```python
from build123d import *

# Parameters (mm, degrees)
SKETCH1_W                       = 150
SKETCH1_H                       = 55
BOSS_EXTRUDE1_DEPTH             = 19.6
SKETCH2_W                       = 27.5
SKETCH2_H                       = 55
BOSS_EXTRUDE2_DEPTH             = 19.6
M8_CLEARANCE_HOLE1_D            = 10
M6_CLEARANCE_HOLE1_D            = 7
FILLET1_R                       = 10
SKETCH11_W                      = 42.4
SKETCH11_H                      = 42.4
CUT_EXTRUDE1_DEPTH              = 10.6
SKETCH13_W                      = 1.8
SKETCH13_H                      = 9
M3_CLEARANCE_HOLE1_AT_2_COUNT   = 2
M3_CLEARANCE_HOLE1_AT_2_PITCH   = 31
M3_CLEARANCE_HOLE1_AT_3_COUNT   = 2
M3_CLEARANCE_HOLE1_AT_3_PITCH   = 43.840620434
M3_CLEARANCE_HOLE1_AT_4_COUNT   = 2
M3_CLEARANCE_HOLE1_AT_4_PITCH   = 31
M3_CLEARANCE_HOLE1_AT_5_COUNT   = 2
M3_CLEARANCE_HOLE1_AT_5_PITCH   = 21.920310217
M3_CLEARANCE_HOLE1_AT_6_COUNT   = 2
M3_CLEARANCE_HOLE1_AT_6_PITCH   = 5
M3_CLEARANCE_HOLE1_AT_7_COUNT   = 2
M3_CLEARANCE_HOLE1_AT_7_PITCH   = 31.400636936
M3_CLEARANCE_HOLE1_AT_8_COUNT   = 2
M3_CLEARANCE_HOLE1_AT_8_PITCH   = 40.459856648
M3_CLEARANCE_HOLE1_AT_9_COUNT   = 2
M3_CLEARANCE_HOLE1_AT_9_PITCH   = 26
M5_CLEARANCE_HOLE1_D            = 5.8
SKETCH17_R                      = 4
CUT_EXTRUDE2_DEPTH              = 108.919692364
SKETCH18_W                      = 0.2
SKETCH18_H                      = 42.4
SKETCH18_W_2                    = 5
SKETCH18_H_2                    = 0.2
CUT_EXTRUDE3_DEPTH              = 10.6
SKETCH19_W                      = 5
SKETCH19_H                      = 5.8
SKETCH19_H_2                    = 3.6
CUT_EXTRUDE4_DEPTH              = 107.652988706
CUT_EXTRUDE5_DEPTH              = 2
SKETCH21_W                      = 12.7
SKETCH21_H                      = 6.35
CUT_EXTRUDE6_DEPTH              = 108.919692364
F_1_4_CLEARANCE_HOLE1_OUTLINE_W = 3.57124
F_1_4_CLEARANCE_HOLE1_OUTLINE_H = 11.625002241


# Read off the part's stored shape, not the designer's step: 1/4 Clearance Hole1
with BuildPart() as part:
    # Sketch1 → Boss-Extrude1 (new body)
    with BuildSketch(Plane(origin=(0, 0, 0), x_dir=(1, 0, 0), z_dir=(0, 1, 0))):
        Rectangle(SKETCH1_W, SKETCH1_H)
    extrude(amount=BOSS_EXTRUDE1_DEPTH)

    # Sketch2 → Boss-Extrude2 (add)
    with BuildSketch(Plane.XZ):
        with Locations((-88.75, 0)):
            Rectangle(SKETCH2_W, SKETCH2_H)
        with BuildLine():
            Line((75, 27.5), (75, -27.5))
            ThreePointArc((75, -27.5), (102.5, 0), (75, 27.5))
        make_face()
    extrude(amount=-BOSS_EXTRUDE2_DEPTH)

    # M8 Clearance Hole1 (through all)
    with Locations(Plane(origin=(0, 0, 0), x_dir=(-1, 0, 0), z_dir=(0, -1, 0))):
        with Locations((-75, 0)):
            Hole(M8_CLEARANCE_HOLE1_D / 2)

    # M6 Clearance Hole1 (through all)
    with Locations(Plane(origin=(0, 19.6, 0), x_dir=(1, 0, 0), z_dir=(0, 1, 0))):
        with Locations((62, 0), (88, 0)):
            Hole(M6_CLEARANCE_HOLE1_D / 2)

    # Fillet1
    fillet1_edges = [part.edges().sort_by_distance(p)[0] for p in [
        (-102.5, 9.8, -27.5),
        (-102.5, 9.8, 27.5),
    ]]
    fillet(fillet1_edges, radius=FILLET1_R)

    # Sketch11 → Cut-Extrude1 (cut)
    with BuildSketch(Plane.XZ):
        with Locations((-10, 0)):
            Rectangle(SKETCH11_W, SKETCH11_H)
    extrude(amount=-CUT_EXTRUDE1_DEPTH, mode=Mode.SUBTRACT)

    # Sketch13 → M3 Clearance Hole1 (revolve, cut)
    with BuildSketch(Plane(origin=(5.5, 10.6, -15.5), x_dir=(0, 0, -1), z_dir=(1, 0, 0))):
        with Locations((0.9, 4.5)):
            Rectangle(SKETCH13_W, SKETCH13_H)
    m3_clearance_hole1 = revolve(axis=Axis((5.5, 4.25, -15.5), (0, 1, 0)), mode=Mode.SUBTRACT)

    # M3 Clearance Hole1 at 2: M3 Clearance Hole1 ×2
    with Locations(*[(-i * M3_CLEARANCE_HOLE1_AT_2_PITCH, 0, 0) for i in range(1, M3_CLEARANCE_HOLE1_AT_2_COUNT)]):
        add(m3_clearance_hole1, mode=Mode.SUBTRACT)

    # M3 Clearance Hole1 at 3: M3 Clearance Hole1 ×2
    with Locations(*[Vector(-0.7071067811865476, 0, 0.7071067811865476) * (i * M3_CLEARANCE_HOLE1_AT_3_PITCH) for i in range(1, M3_CLEARANCE_HOLE1_AT_3_COUNT)]):
        add(m3_clearance_hole1, mode=Mode.SUBTRACT)

    # M3 Clearance Hole1 at 4: M3 Clearance Hole1 ×2
    with Locations(*[(0, 0, i * M3_CLEARANCE_HOLE1_AT_4_PITCH) for i in range(1, M3_CLEARANCE_HOLE1_AT_4_COUNT)]):
        add(m3_clearance_hole1, mode=Mode.SUBTRACT)

    # M3 Clearance Hole1 at 5: M3 Clearance Hole1 ×2
    with Locations(*[Vector(-0.7071067811865476, 0, 0.7071067811865476) * (i * M3_CLEARANCE_HOLE1_AT_5_PITCH) for i in range(1, M3_CLEARANCE_HOLE1_AT_5_COUNT)]):
        add(m3_clearance_hole1, mode=Mode.SUBTRACT)

    # M3 Clearance Hole1 at 6: M3 Clearance Hole1 ×2
    with Locations(*[(i * M3_CLEARANCE_HOLE1_AT_6_PITCH, 0, 0) for i in range(1, M3_CLEARANCE_HOLE1_AT_6_COUNT)]):
        add(m3_clearance_hole1, mode=Mode.SUBTRACT)

    # M3 Clearance Hole1 at 7: M3 Clearance Hole1 ×2
    with Locations(*[Vector(0.15923243882462054, 0, 0.9872411207126471) * (i * M3_CLEARANCE_HOLE1_AT_7_PITCH) for i in range(1, M3_CLEARANCE_HOLE1_AT_7_COUNT)]):
        add(m3_clearance_hole1, mode=Mode.SUBTRACT)

    # M3 Clearance Hole1 at 8: M3 Clearance Hole1 ×2
    with Locations(*[Vector(-0.6426122619764711, 0, 0.7661915431257925) * (i * M3_CLEARANCE_HOLE1_AT_8_PITCH) for i in range(1, M3_CLEARANCE_HOLE1_AT_8_COUNT)]):
        add(m3_clearance_hole1, mode=Mode.SUBTRACT)

    # M3 Clearance Hole1 at 9: M3 Clearance Hole1 ×2
    with Locations(*[(-i * M3_CLEARANCE_HOLE1_AT_9_PITCH, 0, 0) for i in range(1, M3_CLEARANCE_HOLE1_AT_9_COUNT)]):
        add(m3_clearance_hole1, mode=Mode.SUBTRACT)

    # M5 Clearance Hole1 (through all)
    with Locations(Plane(origin=(0, 10.6, 0), x_dir=(-1, 0, 0), z_dir=(0, -1, 0))):
        with Locations((10, 0), (5, 0)):
            Hole(M5_CLEARANCE_HOLE1_D / 2)

    # Sketch17 → Cut-Extrude2 (cut, through all)
    with BuildSketch(Plane.XZ):
        with Locations(Location((-82.5, 0, 0), (0, 0, 270))):
            Circle(SKETCH17_R)
    extrude(amount=-CUT_EXTRUDE2_DEPTH, mode=Mode.SUBTRACT)

    # Sketch18 → Cut-Extrude3 (cut)
    with BuildSketch(Plane.XZ):
        with Locations((-31.3, 0)):
            Rectangle(SKETCH18_W, SKETCH18_H)
        Polygon((11.2, -21.2), (-31.2, -21.2), (-31.4, -21.2), (-31.4, -21.4), (11.2, -21.4), align=None)
        with Locations((13.7, -21.3)):
            Rectangle(SKETCH18_W_2, SKETCH18_H_2)
        Polygon((11.2, 21.4), (11.2, 21.2), (11.2, -21.2), (16.2, -21.2), (16.2, 21.4), align=None)
        Polygon((-31.4, 21.2), (-31.2, 21.2), (11.2, 21.2), (11.2, 21.4), (-31.4, 21.4), align=None)
    extrude(amount=-CUT_EXTRUDE3_DEPTH, mode=Mode.SUBTRACT)

    # Sketch19 → Cut-Extrude4 (cut, through all)
    with BuildSketch(Plane.XZ.offset(-10.6)):
        with BuildLine():
            ThreePointArc((-20.5, 13.7), (-22.3, 15.5), (-20.5, 17.3))
            Line((-20.5, 17.3), (-25.5, 17.3))
            ThreePointArc((-25.5, 17.3), (-24.227207794, 16.772792206), (-23.7, 15.5))
            ThreePointArc((-23.7, 15.5), (-24.227207794, 14.227207794), (-25.5, 13.7))
            Line((-25.5, 13.7), (-20.5, 13.7))
        make_face()
        with BuildLine():
            ThreePointArc((10.5, 13.7), (8.7, 15.5), (10.5, 17.3))
            Line((10.5, 17.3), (5.5, 17.3))
            ThreePointArc((5.5, 17.3), (6.772792206, 16.772792206), (7.3, 15.5))
            ThreePointArc((7.3, 15.5), (6.772792206, 14.227207794), (5.5, 13.7))
            Line((5.5, 13.7), (10.5, 13.7))
        make_face()
        with Locations((-7.5, 0)):
            Rectangle(SKETCH19_W, SKETCH19_H)
        with Locations((8, -15.5)):
            Rectangle(SKETCH19_W, SKETCH19_H_2)
        with Locations((-23, -15.5)):
            Rectangle(SKETCH19_W, SKETCH19_H_2)
    extrude(amount=-CUT_EXTRUDE4_DEPTH, mode=Mode.SUBTRACT)

    # Sketch16 → Cut-Extrude5 (cut)
    with BuildSketch(Plane.XZ.offset(-10.6)):
        with BuildLine():
            Line((-10, 11.2), (-5, 11.2))
            ThreePointArc((-5, 11.2), (6.2, 0), (-5, -11.2))
            Line((-5, -11.2), (-10, -11.2))
            ThreePointArc((-10, -11.2), (-21.2, 0), (-10, 11.2))
        make_face()
    extrude(amount=-CUT_EXTRUDE5_DEPTH, mode=Mode.SUBTRACT)

    # Sketch21 → Cut-Extrude6 (cut, through all)
    with BuildSketch(Plane(origin=(0, 19.6, 0), x_dir=(1, 0, 0), z_dir=(0, 1, 0))):
        with Locations((75, 12.7)):
            Rectangle(SKETCH21_W, SKETCH21_H)
    extrude(amount=-CUT_EXTRUDE6_DEPTH, mode=Mode.SUBTRACT)

    # 1/4 Clearance Hole1 outline → 1/4 Clearance Hole1 (revolve, cut)
    with BuildSketch(Plane(origin=(75, 9.8, 0), x_dir=(1, 0, 0), z_dir=(0, -1, 0))):
        Polygon((2.477440343, -4.342778861), (0, -4.342778861), (0, -9.525), (3.57124, -9.525), (3.571240952, -5.000000572), align=None)
        with Locations((1.78562, -21.687501121)):
            Rectangle(F_1_4_CLEARANCE_HOLE1_OUTLINE_W, F_1_4_CLEARANCE_HOLE1_OUTLINE_H)
    revolve(axis=Axis((75, 9.8, 0), (0, 0, 1)), mode=Mode.SUBTRACT)


solid = part.part
```
Here's how the part is built. I have some questions about the finished solid (model axes, mm). A direction names the side the tool comes from. Coordinates: 2 decimals unless noted, no trailing zeros. Write each loop counter-clockwise with the first axis right and the second up, starting at its lowest first coordinate (ties: lowest second). Pieces come first, ordered by that corner, then holes. Notation, with made-up numbers: (-25, -25.75) - (-1, -25.75) arc R22 ccw to (-1, 6.25) - close; hole circle Ø8 at (1, -37.75). An arc over 180 degrees is marked (long way). One line per item, written item: value.
1) We'd pull the mould along Z, two halves only. Please class faces 5 (the cylindrical face through (-27.3, 15.2, -15.5)), 6 (the flat face through (-102.5, 10, 0)), 7 (the cylindrical face through (102.493, 9.663, -0.605)): pulls with the +Z half, pulls with the -Z half, needs draft (parallel to the pull), parting line crosses it, or undercut.
Model answer:
face 5: undercut
face 6: needs draft
face 7: parting line crosses it
2) Suppose I cut it at C-C on z = 0. State how many separate pieces and enclosed holes the cut face has, and give its area (3 significant figures).
Model answer:
separate pieces: 6
enclosed holes: 0
area: 2,760 mm²
3) I'm going to push flat-ended pins straight in: P1, Ø3, axis at y = 7.5, z = -0.5, coming from the +X side; P2, Ø24.5, axis at x = -11, z = 2, coming from the -Y side; P3, Ø1.9, axis at y = 7.5, z = -11, coming from the +X side; P4, Ø3, axis at x = 51, z = -2.5, coming from the -Y side. Where does each tip first touch, or does it pass through?
Model answer:
P1: stops at x = 102.5
P2: stops at y = 10.6
P3: stops at x = 100.6
P4: stops at y = 0
4) I need wall thicknesses on line 1 along Z through (x, y) = (8.5, 13.25); line 2 along Y through (x, z) = (75, -6.15); line 3 along X through (y, z) = (10.5, -15). Which ranges of each line are inside material? Lowest first, please.
Model answer:
line 1: z = -27.5 to -17.3, -13.7 to 13.7, 17.3 to 27.5
line 2: y = 0 to 6.23, 13.37 to 19.6
line 3: x = -102.5 to -31.4, 16.2 to 68.65, 81.35 to 98.05
5) Suppose I cut it at A-A on x = 62. Write out the boundary of the cut face in (y, z), and give its area (3 significant figures).
Model answer:
outline: (0, -27.5) - (19.6, -27.5) - (19.6, -3.5) - (0, -3.5) - close; (0, 3.5) - (19.6, 3.5) - (19.6, 27.5) - (0, 27.5) - close
area: 941 mm²
6) Suppose I cut it at B-B on y = 3. Write out the boundary of the cut face in (x, z) (3 decimals).
Model answer:
outline: (-102.5, -17.5) arc R10 ccw to (-92.5, -27.5) - (75, -27.5) arc R27.5 ccw to (75, 27.5) - (-92.5, 27.5) arc R10 ccw to (-102.5, 17.5) - close; hole circle Ø8 at (-82.5, 0); hole (-31.4, -21.4) - (16.2, -21.4) - (16.2, 21.4) - (-31.4, 21.4) - close; hole circle Ø7 at (62, 0); hole (68.65, -15.875) - (81.35, -15.875) - (81.35, -9.525) - (68.65, -9.525) - close; hole circle Ø10 at (75, 0); hole circle Ø7 at (88, 0)
7) On a 3-axis mill with a long thin cutter (end or side, diameter ignored), from which of +Z, -Z, +X, -X, +Y, -Y can I reach the whole of each face in a straight line? I mean faces 1 (the flat face through (-1, 0, -24)), 2 (the conical face through (72.348, 9.858, -4.448)), 3 (the cylindrical face through (12.3, 15.2, 15.5)), 4 (the flat face through (-7, 12.6, -5)). Say none if no direction works.
Model answer:
face 1: +Z, -Z, +X, -X, -Y
face 2: -Z
face 3: +Y, -Y
face 4: -Y
